from build123d import *

# Parameters (mm, degrees)
F1_DEPTH = 1.5
F2_R     = 13.7922
F3_DEPTH = 25.4
F5_DEPTH = 25.4
F8_DEPTH = 1.4732


# Not quite as in the source:
# - a variable given as a bare number and used for a length is read in inches; the dataset says mm whatever the document's units were


with BuildPart() as f1:
    # F0 (on Front) → F1 (new body)
    with BuildSketch(Plane.XZ):
        with BuildLine():
            ThreePointArc((-27.5336, 15.24), (-38.3099073453, -10.7763073453), (-12.2936, 0))
            ThreePointArc((-12.2936, 0), (-12.9572083605, 4.4481914045), (-14.8902413086, 8.509))
            ThreePointArc((-14.8902413086, 8.509), (-20.3718809326, 13.4524116797), (-27.5336, 15.24))
        make_face()
        with BuildLine():
            ThreePointArc((-27.5336, 15.24), (-20.3718809326, 13.4524116797), (-14.8902413086, 8.509))
            Line((-14.8902413086, 8.509), (14.8902413086, 8.509))
            ThreePointArc((14.8902413086, 8.509), (20.3718809326, 13.4524116797), (27.5336, 15.24))
            Line((27.5336, 15.24), (-27.5336, 15.24))
        make_face()
        with BuildLine():
            ThreePointArc((27.5336, 15.24), (20.3718809326, 13.4524116797), (14.8902413086, 8.509))
            ThreePointArc((14.8902413086, 8.509), (23.0854085955, -14.5763916395), (42.7736, 0))
            ThreePointArc((42.7736, 0), (38.3099073453, 10.7763073453), (27.5336, 15.24))
        make_face()
    extrude(amount=F1_DEPTH)

    # F2 (on face) → F3 (cut)
    with BuildSketch(Plane.XZ.offset(1.5)):
        with Locations((-27.5336, 0)):
            Circle(F2_R)
        with Locations((27.5336, 0)):
            Circle(F2_R)
        with BuildLine():
            Line((0, 40.3644442558), (-21.547392987, 18.4778384864))
            Line((-21.547392987, 18.4778384864), (-16.5919354635, 13.522380963))
            ThreePointArc((-16.5919354635, 13.522380963), (-14.2228731292, 11.9602304674), (-11.43, 11.4576071501))
            Line((-11.43, 11.4576071501), (0, 11.4576071501))
            Line((0, 11.4576071501), (0, 40.3644442558))
        make_face()
        with BuildLine():
            Line((21.547392987, 18.4778384864), (0, 40.3644442558))
            Line((0, 40.3644442558), (0, 11.4576071501))
            Line((0, 11.4576071501), (11.43, 11.4576071501))
            ThreePointArc((11.43, 11.4576071501), (14.2228731292, 11.9602304674), (16.5919354635, 13.522380963))
            Line((16.5919354635, 13.522380963), (21.547392987, 18.4778384864))
        make_face()
    extrude(amount=-F3_DEPTH, mode=Mode.SUBTRACT)

    # F4 (on face) → F5 (cut)
    with BuildSketch(Plane.XZ.offset(1.5)):
        Polygon((-9.2328525533, 17.0485330061), (-24.6466696262, 16.6515540332), (-11.43, 11.4576071501), align=None)
        Polygon((11.43, 11.4576071501), (24.6466696262, 16.6515540332), (9.2328525533, 17.0485330061), align=None)
    extrude(amount=-F5_DEPTH, mode=Mode.SUBTRACT)

    # F7 (on Front) → F8 (join)
    with BuildSketch(Plane.XZ):
        with BuildLine():
            ThreePointArc((-17.6120530814, 10.0212339312), (-15.0131826274, 7.0473877292), (-13.4240113708, 3.4318070584))
            ThreePointArc((-13.4240113708, 3.4318070584), (-7.9783410744, 5.4701683575), (-2.5081751928, 7.4418496173))
            ThreePointArc((-2.5081751928, 7.4418496173), (-1.2673351307, 7.7068584172), (0, 7.6454142109))
            ThreePointArc((0, 7.6454142109), (1.2673351307, 7.7068584172), (2.5081751928, 7.4418496173))
            ThreePointArc((2.5081751928, 7.4418496173), (7.9783410744, 5.4701683575), (13.4240113708, 3.4318070584))
            ThreePointArc((13.4240113708, 3.4318070584), (15.0131826274, 7.0473877292), (17.6120530814, 10.0212339312))
            Line((17.6120530814, 10.0212339312), (-17.6120530814, 10.0212339312))
        make_face()
    extrude(amount=F8_DEPTH)


solid = f1.part
CAD build for the part. Positions are in the model's coordinates, mm. A direction names the side the tool comes from. Round coordinates to 2 decimals unless told otherwise and drop trailing zeros. Order: outer loops, then holes, each group sorted by start corner. A loop starts at its lowest first (then second) coordinate and runs counter-clockwise, first axis right, second up. Notation, with made-up numbers: M -39,17 L -34,17 A10 cw -34,23 Z; hole C 72.5,37 d4. An arc over 180 degrees is marked long. Use one line per item in the form item = value.
Q1. Two-plate mould, pull along X, no slides. Class faces 1 (the flat face through (-3, 0, 8)), 2 (the cylindrical face through (7.57, -0.73, 5.62)): +X half, -X half, draft (parallel to the pull), parting line (faces both ways), or undercut.
Recorded:
face_1 = draft
face_2 = undercut
Q2. Saw through at A-A on x = -36.5. Give the cut face in (y, z).
Recorded:
outline = M -1.5,-12.32 L 0,-12.32 L 0,-10.48 L -1.5,-10.48 Z; M -1.5,10.48 L 0,10.48 L 0,12.32 L -1.5,12.32 Z
Q3. Probe L1, parallel to Z at x = -27.5, y = -1.3; L2, parallel to X at y = -1.2, z = -8; L3, parallel to X at y = -0.85, z = -10. List the from-to ranges inside material, lowest first.
Recorded:
L1 = -15.24 to -13.79, 13.79 to 15.24
L2 = -40.51 to -38.77, -16.3 to -14.56, 14.56 to 16.3, 38.77 to 40.51
L3 = -39.03 to -37.03, -18.03 to -16.03, 16.03 to 18.03, 37.03 to 39.03
Q4. Saw through at D-D on z = 5. State how many separate pieces and enclosed holes the cut face has, then the cut area to 3 significant figures.
Recorded:
separate_pieces = 4
enclosed_holes = 0
area = 20.7 mm^2
Q5. Saw through at C-C on y = -0.4. Give the cut face in (x, z).
Recorded:
outline = M -27.53,15.24 A15.24 ccw long -12.75,3.69 A475.95 cw -2.51,7.44 A4.92 cw 0,7.65 A4.92 cw 2.51,7.44 A475.95 cw 12.75,3.69 A15.24 ccw long 27.53,15.24 L 21.05,15.24 L 16.53,13.46 A7.06 cw 11.43,11.46 L -11.43,11.46 A7.06 cw -16.53,13.46 L -21.05,15.24 Z; hole C -27.53,0 d27.58; hole C 27.53,0 d27.58
Q6. Saw through at B-B on z = 1. Give the cut face in (x, y).
Recorded:
outline = M -42.74,-1.5 L -41.29,-1.5 L -41.29,0 L -42.74,0 Z; M -13.78,-1.5 L -12.33,-1.5 L -12.33,0 L -13.78,0 Z; M 12.33,-1.5 L 13.78,-1.5 L 13.78,0 L 12.33,0 Z; M 41.29,-1.5 L 42.74,-1.5 L 42.74,0 L 41.29,0 Z
Q7. Which spindle directions (+Z, -Z, +X, -X, +Y, -Y) get a long thin tool onto all of the face, cutting with end or side? Do faces 3 (the flat face through (0, -1, 11.458)), 4 (the cylindrical face through (-21.169, -0.76, -12.236)). Say none if no direction does.
Recorded:
face_3 = +Z, +Y, -Y
face_4 = +Y, -Y
